Solid Edge part; units mm, degrees
sketch "Sketch1" plane through (0, 0, 0) normal (0, -1, 0) x (1, 0, 0)
  line L0 (-20.25, 28.5) -> (-20.25, 0)
  line L1 (-20.25, 0) -> (20.25, 0)
  line L2 (20.25, 0) -> (20.25, 28.5)
  line L3 (20.25, 28.5) -> (27.25, 28.5)
  line L4 (27.25, 28.5) -> (27.25, 31)
  line L5 (27.25, 31) -> (20.25, 31)
  line L6 (20.25, 31) -> (20.25, 36.75)
  line L7 (20.25, 36.75) -> (14.55, 36.75)
  line L8 (14.55, 36.75) -> (14.55, 39.25)
  line L9 (14.55, 39.25) -> (-14.55, 39.25)
  line L10 (-14.55, 39.25) -> (-14.55, 36.75)
  line L11 (-14.55, 36.75) -> (-20.25, 36.75)
  line L12 (-20.25, 36.75) -> (-20.25, 31)
  line L13 (-20.25, 31) -> (-27.25, 31)
  line L14 (-27.25, 31) -> (-27.25, 28.5)
  line L15 (-27.25, 28.5) -> (-20.25, 28.5)
  dimension "D1" = 27.25
extrude "Protrusion1" add sketch "Sketch1" along normal mid plane 20
hole "Hole_1" at (25.25, 5, 31) direction (0, 0, -1) diameter 4.25 end up to next
hole "Hole1" at (25.25, -5, 31) direction (0, 0, -1) diameter 4.25 end up to next
sketch "Sketch2" plane through (0, 0, 0) normal (0, -1, 0) x (1, 0, 0)
  line L0 (-20.25, 36.75) -> (-10.25, 36.75)
  line L1 (-10.25, 36.75) -> (-10.25, 41.15)
  line L2 (-10.25, 41.15) -> (-15.65, 41.15)
  line L3 (-15.65, 41.15) -> (-15.65, 40.65)
  line L4 (-15.65, 40.65) -> (-16.85, 40.65)
  line L5 (-16.85, 40.65) -> (-16.85, 39.25)
  line L6 (-16.85, 39.25) -> (-20.25, 39.25)
  line L7 (-20.25, 39.25) -> (-20.25, 36.75)
  dimension "D1" = 10.25
  dimension "D2" = 16.85
  dimension "D3" = 15.65
revolve "RevolvedProtrusion1" add sketch "Sketch2" angle 360 about axis through (-10.25, 0, 50) along (0, 0, -1)
sketch "Sketch3" plane through (-20.25, 0, 14.25) normal (-1, 0, 0) x (0, -1, 0)
  line L0 (-4, -10.25) -> (4, -10.25)
  line L1 (4, -10.25) -> (4, -6.25)
  line L2 (4, -6.25) -> (-4, -6.25)
  line L3 (-4, -6.25) -> (-4, -10.25)
  dimension "D1" = 4
  dimension "D2" = 4
extrude "ExtrudedProtrusion_2" add sketch "Sketch3" along normal blind 2.5
sketch "Sketch4" plane through (-10.25, 0, 41.15) normal (0, 0, 1) x (1, 0, 0)
  arc A0 (-4.3, 9.0283) -> (0, 10) centre (0, 0) cw
  line L0 (-4.3, 10) -> (0, 10)
  line L1 (-4.3, 9.0283) -> (-4.3, 10)
  arc A1 (-4.3, -9.0283) -> (0, -10) centre (0, 0) ccw
  line L2 (-4.3, -10) -> (0, -10)
  line L3 (-4.3, -9.0283) -> (-4.3, -10)
extrude "Cutout1" cut sketch "Sketch4" against normal up to vertex (4.4 mm away)
hole "Hole_3" at (-10.25, 0, 41.15) direction (0, 0, -1) diameter 6 depth 20 tip angle 118
chamfer "Chamfer_1" distance 1 angle 45 4 edges at (-20.25, 0, 0) (0, -10, 0) (20.25, 0, 0) (0, 10, 0)
sketch "Sketch5" plane through (23.75, 0, 31) normal (0, 0, 1) x (-1, 0, 0)
  line L0 (3.5, -0.5) -> (3.5, 0.5)
  line L1 (3.5, 0.5) -> (-3.5, 0.5)
  line L2 (-3.5, 0.5) -> (-3.5, -0.5)
  line L3 (-3.5, -0.5) -> (3.5, -0.5)
  dimension "D1" = 3.5
extrude "ExtrudedProtrusion_3" add sketch "Sketch5" along normal blind 1
mirror "Mirror1" about plane through (0, 0, 0) normal (1, 0, 0) of "Hole_1", "Hole1", "ExtrudedProtrusion_3"
properties material "ABS Plastic, medium impact"
Read the model definition and answer for the solid it produces. Units are mm, in the model's axes. A direction names the side the tool comes from. Round coordinates to 2 decimals unless told otherwise and drop trailing zeros. Order: outer loops, then holes, each group sorted by start corner. A loop starts at its lowest first (then second) coordinate and runs counter-clockwise, first axis right, second up.
1) The part is cut by section B-B on z = 22. Write down the section's boundary in (x, y), plus the area to 3 significant figures.
2) The part is cut by section C-C on y = 8. Write down the section's boundary in (x, z), plus the area to 3 significant figures.
3) Straight lines are drawn through the part: L1, parallel to Y at x = -25.25, z = 30.15 (3 decimals); L2, parallel to Y at x = -10, z = 27; L3, parallel to X at y = 3.5, z = 29.5. For each, find the intervals that lie inside material, in ascending order.
4) For faces 5 (the face through (14.55, 0, 38)), 6 (the face through (23, -6, 31)), 7 (the face through (20.25, 0, 15)), determine the directions among +Z, -Z, +X, -X, +Y, -Y from which every point of the face is accessible in a straight line to the end or side of a thin tool.
5) The mould has two halves that part along Z. Classify faces 1 (the face through (-13, -2, 41.15)), 2 (the face through (-20.25, 0, 34)), 3 (the face through (-21, 0, 8)), 4 (the face through (-20.25, 0, 15)): released by +Z, released by -Z, zero draft, split by the parting line, or undercut.
6) Flat-ended cylindrical pins translate along their axes: pin 1 (12 mm diameter, centred on x = 5.5, y = 0.5, fed in from +Z); pin 2 (1.2 mm diameter, centred on x = -21, y = 0, fed in from +Z); pin 3 (3.5 mm diameter, centred on x = -25, y = -7.5, fed in from +Z). Find the tip coordinate at first contact, or state that the pin passes through.
7) The part is cut by section D-D on x = -1.5. Write down the section's boundary in (y, z).
8) The part is cut by section A-A on x = -25.25. Write down the section's boundary in (y, z) (3 decimals), plus the area to 4 significant figures.
Resolved:
1. outline: (-20.25, -10) - (20.25, -10) - (20.25, 10) - (-20.25, 10) - close; hole circle Ø6 at (-10.25, 0)
1. area: 782 mm2
2. outline: (-27.25, 28.5) - (-20.25, 28.5) - (-20.25, 1) - (-19.25, 0) - (19.25, 0) - (20.25, 1) - (20.25, 28.5) - (27.25, 28.5) - (27.25, 31) - (20.25, 31) - (20.25, 36.75) - (14.55, 36.75) - (14.55, 39.25) - (-16.25, 39.25) - (-16.25, 36.75) - (-20.25, 36.75) - (-20.25, 31) - (-27.25, 31) - close
2. area: 1,600 mm2
3. L1: y = -10 to -7.125, -2.875 to 2.875, 7.125 to 10
3. L2: y = -10 to -2.99, 2.99 to 10
3. L3: x = -27.25 to -26.76, -23.74 to 23.74, 26.76 to 27.25
4. face 5: +Z, +X, +Y, -Y
4. face 6: +Z, +X, -Y
4. face 7: -Z, +X, +Y, -Y
5. face 1: released by +Z
5. face 2: zero draft
5. face 3: undercut
5. face 4: undercut
6. pin 1: stops at z = 39.25
6. pin 2: stops at z = 32
6. pin 3: stops at z = 31
7. outline: (-10, 1) - (-9, 0) - (9, 0) - (10, 1) - (10, 39.25) - (-10, 39.25) - close
8. outline: (-10, 28.5) - (-7.125, 28.5) - (-7.125, 31) - (-10, 31) - close; (-2.875, 28.5) - (2.875, 28.5) - (2.875, 31) - (0.5, 31) - (0.5, 32) - (-0.5, 32) - (-0.5, 31) - (-2.875, 31) - close; (7.125, 28.5) - (10, 28.5) - (10, 31) - (7.125, 31) - close
8. area: 29.75 mm2
